from build123d import *

# Parameters (mm, degrees)
SKETCH1_R           = 3.5
SKETCH1_R_2         = 2.5
BOSS_EXTRUDE1_DEPTH = 4
BOSS_EXTRUDE2_DEPTH = 2


with BuildPart() as part:
    # Sketch1 → Boss-Extrude1 (new body)
    with BuildSketch(Plane(origin=(0, 0, 0), x_dir=(1, 0, 0), z_dir=(0, 1, 0))):
        with Locations(Location((0, 0, 0), (0, 0, 270))):
            Circle(SKETCH1_R)
        with Locations(Location((0, 0, 0), (0, 0, 270))):
            Circle(SKETCH1_R_2, mode=Mode.SUBTRACT)
    extrude(amount=BOSS_EXTRUDE1_DEPTH)

    # Sketch2 → Boss-Extrude2 (add)
    with BuildSketch(Plane(origin=(0, 0, 0), x_dir=(1, 0, 0), z_dir=(0, 1, 0))):
        with BuildLine():
            Line((-2.5, 2.449489743), (-2.5, 7.5))
            ThreePointArc((-2.5, 7.5), (0, 10), (2.5, 7.5))
            Line((2.5, 7.5), (2.5, 2.449489743))
            ThreePointArc((2.5, 2.449489743), (0, 3.5), (-2.5, 2.449489743))
        make_face()
        with BuildLine():
            Line((2.5, 4.5), (2.5, 0))
            Line((2.5, 0), (2.5, -4.5))
            Line((2.5, -4.5), (18.315318835, -1.974987097))
            ThreePointArc((18.315318835, -1.974987097), (20, 0), (18.315318835, 1.974987097))
            Line((18.315318835, 1.974987097), (2.5, 4.5))
        make_face()
        with BuildLine():
            Line((-2.5, -2.449489743), (-2.5, -7.5))
            ThreePointArc((-2.5, -7.5), (0, -10), (2.5, -7.5))
            Line((2.5, -7.5), (2.5, -2.449489743))
            ThreePointArc((2.5, -2.449489743), (0, -3.5), (-2.5, -2.449489743))
        make_face()
        with BuildLine():
            Line((-2.5, -4), (-2.5, 0))
            Line((-2.5, 0), (-2.5, 4))
            Line((-2.5, 4), (-16.290032176, 1.978858594))
            ThreePointArc((-16.290032176, 1.978858594), (-18, 0), (-16.290032176, -1.978858594))
            Line((-16.290032176, -1.978858594), (-2.5, -4))
        make_face()
    extrude(amount=BOSS_EXTRUDE2_DEPTH)


solid = part.part
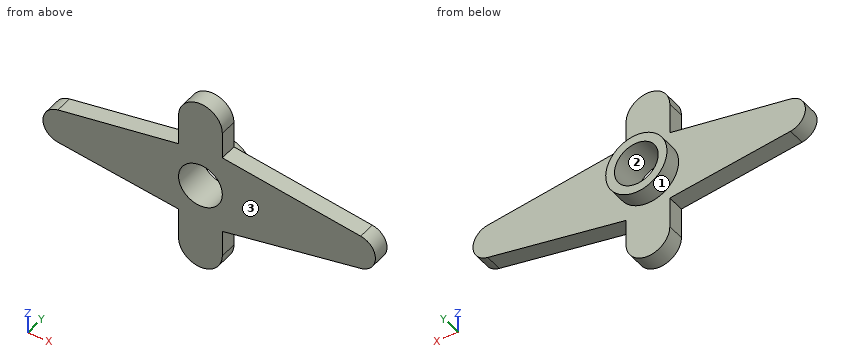
Geometry check sheet. Reference: the model listing, model coordinates, mm. Face numbers are marked on the shaded views. Coordinates: 2 decimals unless noted, no trailing zeros. Write each loop counter-clockwise with the first axis right and the second up, starting at its lowest first coordinate (ties: lowest second). Pieces come first, ordered by that corner, then holes. Notation, with made-up numbers: (-36, -20) -> (-15, -20) arc R18 ccw to (-15, -16) -> close; hole circle Ø5 at (59.25, 38.5). An arc over 180 degrees is marked (long way). One line per question, with ' | ' between items.
1. Depth check by flat-ended pin: pin 1 Ø0.6 at (y, z) = (0.5, 6) entering from +X; pin 2 Ø5 at (x, z) = (13.5, 6.5) entering from +Y; pin 3 Ø1 at (x, z) = (-5, -2.5) entering from +Y; pin 4 Ø0.6 at (y, z) = (1, -5.5) entering from -X. Enter the tip coordinate at first touch or a pass-through.
Answers:
pin 1: stops at x = 2.5 | pin 2: passes through | pin 3: stops at y = 2 | pin 4: stops at x = -2.5
2. Cross-section at A-A on x = 0. Record the cut outline in (y, z).
Answers:
outline: (0, -10) -> (2, -10) -> (2, -3.5) -> (4, -3.5) -> (4, -2.5) -> (0, -2.5) -> close; (0, 2.5) -> (4, 2.5) -> (4, 3.5) -> (2, 3.5) -> (2, 10) -> (0, 10) -> close
3. Cross-section at D-D on z = -5.5. Record the cut outline in (x, y), and give its area (3 significant figures).
Answers:
outline: (-2.5, 0) -> (2.5, 0) -> (2.5, 2) -> (-2.5, 2) -> close | area: 10.0 mm²
4. Cross-section at B-B on z = 0. Record the cut outline in (x, y), and give its area (3 significant figures).
Answers:
outline: (-18, 0) -> (-2.5, 0) -> (-2.5, 4) -> (-3.5, 4) -> (-3.5, 2) -> (-18, 2) -> close; (2.5, 0) -> (20, 0) -> (20, 2) -> (3.5, 2) -> (3.5, 4) -> (2.5, 4) -> close | area: 70.0 mm²
5. Cross-section at C-C on y = 0.7. Record the cut outline in (x, z).
Answers:
outline: (-16.29, -1.98) -> (-2.5, -4) -> (-2.5, -7.5) arc R2.5 ccw to (2.5, -7.5) -> (2.5, -4.5) -> (18.32, -1.97) arc R2 ccw to (18.32, 1.97) -> (2.5, 4.5) -> (2.5, 7.5) arc R2.5 ccw to (-2.5, 7.5) -> (-2.5, 4) -> (-16.29, 1.98) arc R2 ccw to start; hole circle Ø5 at (0, 0)
6. Draft check along X on the marked faces 1, 2 and 3. Enter one of: +X half, -X half, draft (parallel to the pull), parting line (faces both ways), or undercut.
Answers:
face 1: parting line | face 2: undercut | face 3: draft
7. Thickness scan on probe 1 along X at (y, z) = (2.5, 0); probe 2 along Z at (x, y) = (0, 1.55); probe 3 along Y at (x, z) = (-0.5, -8.75). Record the ranges inside material, lowest first. Write a range as from..to.
Answers:
probe 1: x = -3.5..-2.5, 2.5..3.5 | probe 2: z = -10..-2.5, 2.5..10 | probe 3: y = 0..2
